from build123d import *

# Parameters (mm, degrees)
SKETCH1_W             = 20
SKETCH1_H             = 20
BOSS_EXTRUDE1_DEPTH   = 100
M5_TAPPED_HOLE1_D     = 4.2
M5_TAPPED_HOLE1_DEPTH = 12.4
M5_TAPPED_HOLE1_TIP   = 1.2618073
M5_TAPPED_HOLE2_D     = 4.2
M5_TAPPED_HOLE2_DEPTH = 12.4
M5_TAPPED_HOLE2_TIP   = 1.2618073


with BuildPart() as part:
    # Sketch1 → Boss-Extrude1 (new body)
    with BuildSketch(Plane(origin=(0, 0, 0), x_dir=(1, 0, 0), z_dir=(0, 1, 0))):
        with Locations((10, 10)):
            Rectangle(SKETCH1_W, SKETCH1_H)
    extrude(amount=BOSS_EXTRUDE1_DEPTH)

    # Sketch5 → M8 Tapped Hole1 (revolve, cut)
    with BuildSketch(Plane(origin=(10, 100, -10), x_dir=(0, 0, 1), z_dir=(1, 0, 0))):
        Polygon((0, 0), (0, 15.792926105), (3.4, 13.75), (3.4, 0), align=None)
    m8_tapped_hole1 = revolve(axis=Axis((10, 106.35, -10), (0, -1, 0)), mode=Mode.SUBTRACT)

    # Mirror1: M8 Tapped Hole1 across plane
    add(m8_tapped_hole1.mirror(Plane.ZX.offset(50)), mode=Mode.SUBTRACT)

    # M5 Tapped Hole1
    with Locations(Plane.XY):
        with Locations((10, 80), (10, 92.5)):
            Hole(M5_TAPPED_HOLE1_D / 2, depth=M5_TAPPED_HOLE1_DEPTH)
            with Locations((0, 0, -(M5_TAPPED_HOLE1_DEPTH + M5_TAPPED_HOLE1_TIP / 2))):  # 118° drill point
                Cone(0, M5_TAPPED_HOLE1_D / 2, M5_TAPPED_HOLE1_TIP, mode=Mode.SUBTRACT)

    # M5 Tapped Hole2
    with Locations(Plane(origin=(20, 0, 0), x_dir=(0, 0, -1), z_dir=(1, 0, 0))):
        with Locations((10, 7.5), (10, 20)):
            Hole(M5_TAPPED_HOLE2_D / 2, depth=M5_TAPPED_HOLE2_DEPTH)
            with Locations((0, 0, -(M5_TAPPED_HOLE2_DEPTH + M5_TAPPED_HOLE2_TIP / 2))):  # 118° drill point
                Cone(0, M5_TAPPED_HOLE2_D / 2, M5_TAPPED_HOLE2_TIP, mode=Mode.SUBTRACT)


solid = part.part
Input: part model. Units: mm. Frame: model coordinates. A direction names the side the tool comes from. Round coordinates to 2 decimals unless told otherwise and drop trailing zeros.
1) Reachability of faces 5 (the cylindrical face through (9.9, 93.2, -13.4)), 6 (the cylindrical face through (13.713, 21.419, -11.548)), 7 (the cylindrical face through (12.1, 92.59, -3.71)) from +Z, -Z, +X, -X, +Y, -Y: full face, straight path, thin tool, end or side. Return the list, or none.
2) Ray query, L1, parallel to Y at x = 14, z = -10; L2, parallel to X at y = 80, z = -9; L3, parallel to Y at x = 10, z = -4.5. Return the intervals inside material, ascending.
3) Draft query along X for faces 1 (the conical face through (9.82, 84.56, -9.44)), 2 (the flat face through (20, 49, -10)), 3 (the flat face through (0, 49, -10)), 4 (the flat face through (14, 100, -10)). Return one class per face: pulls with the +X half, pulls with the -X half, needs draft (parallel to the pull), parting line crosses it, or undercut.
4) Contact query for flat-ended pins moving along their axis: P1, Ø3.5, axis at x = 10, y = 92.5, coming from the +Z side; P2, Ø6, axis at x = 10, z = -10, coming from the +Y side. Output: stop coordinate, or through.
Geometry says:
1. face 5: +Y
1. face 6: +X
1. face 7: +Z
2. L1: y = 0 to 5.4, 9.6 to 17.9, 22.1 to 100
2. L2: x = 0 to 7.9, 12.1 to 20
2. L3: y = 0 to 77.9, 82.1 to 90.4, 94.6 to 100
3. face 1: undercut
3. face 2: pulls with the +X half
3. face 3: pulls with the -X half
3. face 4: needs draft
4. P1: stops at z = -12.92
4. P2: stops at y = 86.01
